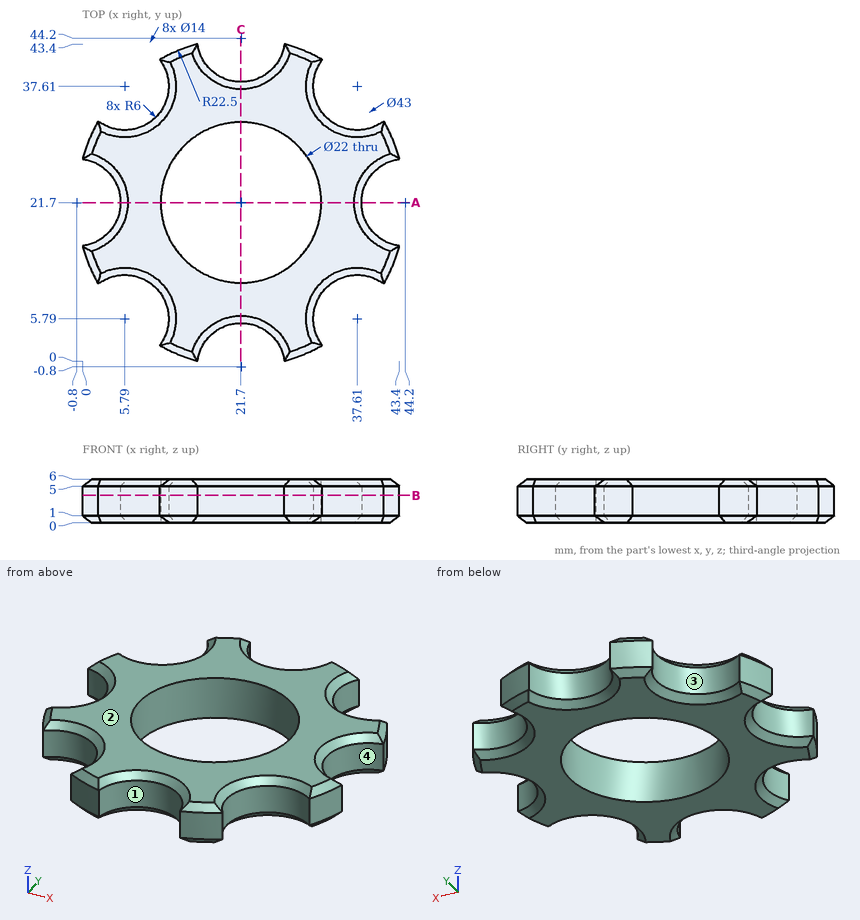
Can you work these out from the drawing? Everything is in mm from the part's minimum corner. Give positions to 0.01 mm unless a question says otherwise; leave off trailing zeros. Order: outer loops, then holes, each group sorted by start corner. A loop starts at its lowest first (then second) coordinate and runs counter-clockwise, first axis right, second up. Notation, with made-up numbers: M 85.5,46 L 144.5,46 A11 ccw 144.5,66 Z; hole C 26.25,55 d1. An arc over 180 degrees is marked long. Use a Markdown table: item, result. Add a question column.
Item 1: Will these pins go through, and if not, where does the flat tip stop? pin 1 (1.5 mm diameter, centred on x = 26, z = 4, fed in from +Y); pin 2 (6 mm diameter, centred on x = 21.5, y = 14.5, fed in from -Z); pin 3 (3 mm diameter, centred on y = 29.5, z = 2, fed in from -X).
Item 2: Suppose I cut it at B-B (z = 3.75). List the corners of the cut face in (x, y) for me, then the cut area to 3 significant figures.
Item 3: Suppose I cut it at A-A (y = 21.7). List the corners of the cut face in (x, z) for me, then the cut area to 3 significant figures.
Item 4: We'd pull the mould along X, two halves only. Please class the marked faces 1, 2, 3 and 4: +X half, -X half, draft (parallel to the pull), parting line (faces both ways), or undercut.
Item 5: If I drill on L1, parallel to Y at x = 21.5, z = 3; L2, parallel to X at y = 12, z = 2.25; L3, parallel to Y at x = 22, z = 0.75, over which ranges is the centre line in solid material (lowest first)? Write a range as [from, to].
Answer sheet:
| question | item | result |
|---|---|---|
| 1 | pin 1 | stops at y = 40.96 |
| 1 | pin 2 | passes through |
| 1 | pin 3 | stops at x = 0.1 |
| 2 | outline | M 0,15.75 A22.5 ccw 2.15,10.56 A6 cw 10.56,2.15 A22.5 ccw 15.75,0 A6 cw 27.65,0 A22.5 ccw 32.84,2.15 A6 cw 41.25,10.56 A22.5 ccw 43.4,15.75 A6 cw 43.4,27.65 A22.5 ccw 41.25,32.84 A6 cw 32.84,41.25 A22.5 ccw 27.65,43.4 A6 cw 15.75,43.4 A22.5 ccw 10.56,41.25 A6 cw 2.15,32.84 A22.5 ccw 0,27.65 A6 cw Z; hole C 21.7,21.7 d22 |
| 2 | area | 784 mm² |
| 3 | outline | M 5.2,1 L 6.2,0 L 10.7,0 L 10.7,6 L 6.2,6 L 5.2,5 Z; M 32.7,0 L 37.2,0 L 38.2,1 L 38.2,5 L 37.2,6 L 32.7,6 Z |
| 3 | area | 64.0 mm² |
| 4 | face 1 | undercut |
| 4 | face 2 | draft |
| 4 | face 3 | undercut |
| 4 | face 4 | +X half |
| 5 | L1 | y = [5.2, 10.7], [32.7, 38.2] |
| 5 | L2 | x = [1.4, 16.51], [26.89, 42] |
| 5 | L3 | y = [5.44, 10.7], [32.7, 37.96] |
